from build123d import *

# Parameters (mm, degrees)
SKETCH_1_R          = 5
SKETCH_1_R_2        = 2.8
EXTRUDE_1_DEPTH     = 3
SKETCH_2_R          = 0.5
CUT_EXTRUDE_1_DEPTH = 6.5
SKETCH_3_R          = 0.5
CUT_EXTRUDE_2_DEPTH = 6.5


with BuildPart() as part:
    # 草图1 → 凸台-拉伸1 (new body)
    with BuildSketch(Plane.XY):
        Circle(SKETCH_1_R)
        Circle(SKETCH_1_R_2, mode=Mode.SUBTRACT)
    extrude(amount=EXTRUDE_1_DEPTH)

    # 草图2 → 切除-拉伸1 (cut, symmetric)
    with BuildSketch(Plane(origin=(0, 0, 0), x_dir=(1, 0, 0), z_dir=(0, 1, 0))):
        with Locations((0, -1.5)):
            Circle(SKETCH_2_R)
    extrude(amount=CUT_EXTRUDE_1_DEPTH, both=True, mode=Mode.SUBTRACT)

    # 草图3 → 切除-拉伸2 (cut, symmetric)
    with BuildSketch(Plane(origin=(0, 0, 0), x_dir=(0, 0, -1), z_dir=(1, 0, 0))):
        with Locations((-1.5, 0)):
            Circle(SKETCH_3_R)
    extrude(amount=CUT_EXTRUDE_2_DEPTH, both=True, mode=Mode.SUBTRACT)


solid = part.part
Could you check a few things on this model? Use its own coordinates, in mm. Give positions to 0.01 mm unless a question says otherwise; leave off trailing zeros. Order: outer loops, then holes, each group sorted by start corner. A loop starts at its lowest first (then second) coordinate and runs counter-clockwise, first axis right, second up. Notation, with made-up numbers: (77, 57) -> (113, 57) arc R25 ccw to (113, 71) -> close; hole circle Ø8 at (24, -38.5). An arc over 180 degrees is marked (long way). Return JSON: item names as keys, results as strings.
1. Thinking about a two-plate mould opening in Z: for faces 1 (the flat face through (2.2, -2.2, 0)), 2 (the flat face through (2.2, -2.2, 3)), 3 (the cylindrical face through (0, 4, 2)), which applies, pulls with the +Z half, pulls with the -Z half, needs draft (parallel to the pull), parting line crosses it, or undercut?
Answer list:
{"face 1": "pulls with the -Z half", "face 2": "pulls with the +Z half", "face 3": "undercut"}
2. Imagine slicing it at D-D on y = -3.75. List the corners of the cut face in (x, z) for me, then the cut area to 3 significant figures.
Answer list:
{"outline": "(-3.31, 0) -> (3.31, 0) -> (3.31, 3) -> (-3.31, 3) -> close; hole circle Ø1 at (0, 1.5)", "area": "19.1 mm2"}
3. For pin 1 Ø1 at (x, y) = (-2, 0) entering from +Z, with a flat end and sliding along its axis, tell me the tip position at first contact or that it passes through.
Answer list:
{"pin 1": "passes through"}
4. I need wall thicknesses on line 1 (Z direction, x = 0, y = 4.5); line 2 (Y direction, x = -3, z = 1.4); line 3 (Y direction, x = 2.25, z = 1.4). Which ranges of each line are inside material? Lowest first, please. Write a range as from..to.
Answer list:
{"line 1": "z = 0..1, 2..3", "line 2": "y = -4..-0.49, 0.49..4", "line 3": "y = -4.47..-1.67, 1.67..4.47"}
5. Imagine slicing it at C-C on x = 3. List the corners of the cut face in (y, z) for me, then the cut area to 3 significant figures.
Answer list:
{"outline": "(-4, 0) -> (4, 0) -> (4, 3) -> (-4, 3) -> close; hole circle Ø1 at (0, 1.5)", "area": "23.2 mm2"}
6. Imagine slicing it at A-A on y = 0. List the corners of the cut face in (x, z) for me.
Answer list:
{"outline": "(-5, 0) -> (-2.8, 0) -> (-2.8, 1) -> (-5, 1) -> close; (-5, 2) -> (-2.8, 2) -> (-2.8, 3) -> (-5, 3) -> close; (2.8, 0) -> (5, 0) -> (5, 1) -> (2.8, 1) -> close; (2.8, 2) -> (5, 2) -> (5, 3) -> (2.8, 3) -> close"}
